Work out the finished part from the listing and answer in its coordinate system (mm). A direction names the side the tool comes from. Round coordinates to 2 decimals unless told otherwise and drop trailing zeros. Write each loop counter-clockwise with the first axis right and the second up, starting at its lowest first coordinate (ties: lowest second). Pieces come first, ordered by that corner, then holes. Notation, with made-up numbers: (24.5, -20) - (47.5, -20) arc R6 cw to (47.5, -16) - close; hole circle Ø4 at (3, 15). An arc over 180 degrees is marked (long way). Answer as a JSON object with one key per item and string values.
```python
from build123d import *

# Parameters (mm, degrees)
SKETCH1_W            = 18
SKETCH1_H            = 242.5
BOSS_EXTRUDE2_DEPTH  = 5
SKETCH2_W            = 9
SKETCH2_H            = 5
BOSS_EXTRUDE3_DEPTH  = 5
SKETCH3_W            = 5
SKETCH3_H            = 35
BOSS_EXTRUDE4_DEPTH  = 5
SKETCH4_W            = 5
SKETCH4_H            = 25
BOSS_EXTRUDE5_DEPTH  = 5
SKETCH5_W            = 5
SKETCH5_H            = 55
BOSS_EXTRUDE6_DEPTH  = 37.5
SKETCH6_W            = 10
SKETCH6_H            = 5
BOSS_EXTRUDE7_DEPTH  = 5
SKETCH7_W            = 5
SKETCH7_H            = 8.75
BOSS_EXTRUDE8_DEPTH  = 5
SKETCH8_W            = 10
SKETCH8_H            = 5
BOSS_EXTRUDE9_DEPTH  = 5
SKETCH9_W            = 32.5
SKETCH9_H            = 17.5
BOSS_EXTRUDE10_DEPTH = 5
SKETCH10_W           = 10
SKETCH10_H           = 5
BOSS_EXTRUDE11_DEPTH = 5
SKETCH11_R           = 2.1
CUT_EXTRUDE1_DEPTH   = 5
BOSS_EXTRUDE12_DEPTH = 5
SKETCH13_R           = 2.1
CUT_EXTRUDE2_DEPTH   = 5
BOSS_EXTRUDE13_DEPTH = 5
SKETCH15_W           = 4.2
SKETCH15_H           = 5
SKETCH15_W_2         = 10
SKETCH15_H_2         = 10
CUT_EXTRUDE3_DEPTH   = 10


with BuildPart() as part:
    # Sketch1 → Boss-Extrude2 (new body)
    with BuildSketch(Plane.XY):
        with Locations((-9, 121.25)):
            Rectangle(SKETCH1_W, SKETCH1_H)
    extrude(amount=BOSS_EXTRUDE2_DEPTH)

    # Sketch2 → Boss-Extrude3 (add)
    with BuildSketch(Plane(origin=(0, 242.5, 0), x_dir=(1, 0, 0), z_dir=(0, 1, 0))):
        with Locations((-13.5, -2.5)):
            Rectangle(SKETCH2_W, SKETCH2_H)
    extrude(amount=BOSS_EXTRUDE3_DEPTH)

    # Sketch3 → Boss-Extrude4 (add)
    with BuildSketch(Plane(origin=(0, 0, 0), x_dir=(-1, 0, 0), z_dir=(0, 0, -1))):
        with Locations((20.5, 210)):
            Rectangle(SKETCH3_W, SKETCH3_H)
        with Locations((20.5, 150)):
            Rectangle(SKETCH3_W, SKETCH3_H)
        with Locations((20.5, 90)):
            Rectangle(SKETCH3_W, SKETCH3_H)
        with Locations((20.5, 30)):
            Rectangle(SKETCH3_W, SKETCH3_H)
    extrude(amount=-BOSS_EXTRUDE4_DEPTH)

    # Sketch4 → Boss-Extrude5 (add)
    with BuildSketch(Plane.XY.offset(5)):
        with Locations((2.5, 180)):
            Rectangle(SKETCH4_W, SKETCH4_H)
        with Locations((2.5, 120)):
            Rectangle(SKETCH4_W, SKETCH4_H)
    extrude(amount=-BOSS_EXTRUDE5_DEPTH)

    # Sketch5 → Boss-Extrude6 (add)
    with BuildSketch(Plane(origin=(0, 0, 0), x_dir=(0, 0, -1), z_dir=(1, 0, 0))):
        with Locations((-2.5, 27.5)):
            Rectangle(SKETCH5_W, SKETCH5_H)
    extrude(amount=BOSS_EXTRUDE6_DEPTH)

    # Sketch6 → Boss-Extrude7 (add)
    with BuildSketch(Plane.XY.offset(5)):
        with Locations((25, 57.5)):
            Rectangle(SKETCH6_W, SKETCH6_H)
    extrude(amount=-BOSS_EXTRUDE7_DEPTH)

    # Sketch7 → Boss-Extrude8 (add)
    with BuildSketch(Plane.XY.offset(5)):
        with Locations((2.5, 64.375)):
            Rectangle(SKETCH7_W, SKETCH7_H)
    extrude(amount=-BOSS_EXTRUDE8_DEPTH)

    # Sketch8 → Boss-Extrude9 (add)
    with BuildSketch(Plane.XY.offset(5)):
        with Locations((22.5, -2.5)):
            Rectangle(SKETCH8_W, SKETCH8_H)
    extrude(amount=-BOSS_EXTRUDE9_DEPTH)

    # Sketch9 → Boss-Extrude10 (add)
    with BuildSketch(Plane.XY.offset(5)):
        with Locations((21.25, 68.75)):
            Rectangle(SKETCH9_W, SKETCH9_H)
    extrude(amount=-BOSS_EXTRUDE10_DEPTH)

    # Sketch10 → Boss-Extrude11 (add)
    with BuildSketch(Plane.XY.offset(5)):
        with Locations((22.5, 80)):
            Rectangle(SKETCH10_W, SKETCH10_H)
    extrude(amount=-BOSS_EXTRUDE11_DEPTH)

    # Sketch11 → Cut-Extrude1 (cut)
    with BuildSketch(Plane(origin=(0, 0, 0), x_dir=(-1, 0, 0), z_dir=(0, 0, -1))):
        with Locations((-2.5, 180)):
            Circle(SKETCH11_R)
        with Locations((-2.5, 120)):
            Circle(SKETCH11_R)
    extrude(amount=-CUT_EXTRUDE1_DEPTH, mode=Mode.SUBTRACT)

    # Sketch12 → Boss-Extrude12 (add)
    with BuildSketch(Plane(origin=(0, 0, 0), x_dir=(-1, 0, 0), z_dir=(0, 0, -1))):
        with BuildLine():
            Line((-5, 175.669872981), (-5, 184.330127019))
            ThreePointArc((-5, 184.330127019), (-7.5, 180), (-5, 175.669872981))
        make_face()
        with BuildLine():
            Line((-5, 124.330127019), (-5, 115.669872981))
            ThreePointArc((-5, 115.669872981), (-7.5, 120), (-5, 124.330127019))
        make_face()
    extrude(amount=-BOSS_EXTRUDE12_DEPTH)

    # Sketch13 → Cut-Extrude2 (cut)
    with BuildSketch(Plane.XY.offset(5)):
        with Locations((-20.5, 210)):
            Circle(SKETCH13_R)
        with Locations((-20.5, 90)):
            Circle(SKETCH13_R)
    extrude(amount=-CUT_EXTRUDE2_DEPTH, mode=Mode.SUBTRACT)

    # Sketch14 → Boss-Extrude13 (add)
    with BuildSketch(Plane.XY.offset(5)):
        with BuildLine():
            Line((-23, 214.330127019), (-23, 205.669872981))
            ThreePointArc((-23, 205.669872981), (-25.5, 210), (-23, 214.330127019))
        make_face()
        with BuildLine():
            Line((-23, 85.669872981), (-23, 94.330127019))
            ThreePointArc((-23, 94.330127019), (-25.5, 90), (-23, 85.669872981))
        make_face()
    extrude(amount=-BOSS_EXTRUDE13_DEPTH)

    # Sketch15 → Cut-Extrude3 (cut)
    with BuildSketch(Plane.XY.offset(5)):
        with Locations((0, 2.5)):
            Rectangle(SKETCH15_W, SKETCH15_H)
        with Locations((0, 10)):
            Rectangle(SKETCH15_W_2, SKETCH15_H_2)
    extrude(amount=-CUT_EXTRUDE3_DEPTH, mode=Mode.SUBTRACT)


solid = part.part
```
Item 1: A cutting plane is placed at B-B (y = 90). Write down the section's boundary in (x, z).
Results found:
{"outline": "(-25.5, 0) - (-22.6, 0) - (-22.6, 5) - (-25.5, 5) - close; (-18.4, 0) - (0, 0) - (0, 5) - (-18.4, 5) - close"}
Item 2: A cutting plane is placed at D-D (z = 2.55). Give the number of separate pieces and of enclosed holes in the cut face, and give its area (3 significant figures).
Results found:
{"separate pieces": "1", "enclosed holes": "5", "area": "8,070 mm²"}
Item 3: Consider line 1 along Y through (x, z) = (-20.5, 2.85); line 2 along Y through (x, z) = (19, 1.9); line 3 along X through (y, z) = (10, 1.9). Determine where each line is inside the solid, lowest interval first.
Results found:
{"line 1": "12.5 to 47.5, 72.5 to 87.9, 92.1 to 107.5, 132.5 to 167.5, 192.5 to 207.9, 212.1 to 227.5", "line 2": "-5 to 55, 60 to 82.5", "line 3": "-18 to -5, 5 to 37.5"}
Item 4: Each of these flat-tipped pins is pushed along its axis until it touches: P1, Ø1.5, axis at y = 167.5, z = 3, coming from the +X side; P2, Ø1.5, axis at x = 9.5, z = 1.5, coming from the +Y side; P3, Ø2, axis at x = 2, y = 177, coming from the -Z side; P4, Ø3, axis at x = 3, z = 3.5, coming from the +Y side. Where does it stop, or does it pass through?
Results found:
{"P1": "x = 5", "P2": "y = 77.5", "P3": "z = 0", "P4": "y = 192.5"}
Item 5: For faces 1 (the flat face through (-18, 120, 3)), 2 (the flat face through (32, 77.5, 3)), 3 (the flat face through (-20, 227.5, 2)), 4 (the flat face through (34, 55, 3)), determine the directions among +Z, -Z, +X, -X, +Y, -Y from which every point of the face is accessible in a straight line to the end or side of a thin tool.
Results found:
{"face 1": "+Z, -Z, -X", "face 2": "+Z, -Z, +X, +Y", "face 3": "+Z, -Z, -X, +Y", "face 4": "+Z, -Z, +X"}
Item 6: A cutting plane is placed at A-A (x = 13.5). Write down the section's boundary in (y, z), and give its area (4 significant figures).
Results found:
{"outline": "(0, 0) - (55, 0) - (55, 5) - (0, 5) - close; (60, 0) - (77.5, 0) - (77.5, 5) - (60, 5) - close", "area": "362.5 mm²"}
Item 7: Determine the mould class of faces 5 (the flat face through (-9, 245, 3)), 6 (the flat face through (10, 55, 3)), 7 (the flat face through (-20, 107.5, 2)) for opening direction X: pulls with the +X half, pulls with the -X half, needs draft (parallel to the pull), parting line crosses it, or undercut.
Results found:
{"face 5": "pulls with the +X half", "face 6": "undercut", "face 7": "needs draft"}
Item 8: A cutting plane is placed at C-C (y = 171.5). Write down the section's boundary in (x, z), and give its area (3 significant figures).
Results found:
{"outline": "(-18, 0) - (5, 0) - (5, 5) - (-18, 5) - close", "area": "115 mm²"}
